Can you work these out from the drawing? Everything is in mm from the part's minimum corner. A direction names the side the tool comes from. Coordinates: 2 decimals unless noted, no trailing zeros. Order: outer loops, then holes, each group sorted by start corner. A loop starts at its lowest first (then second) coordinate and runs counter-clockwise, first axis right, second up. Notation, with made-up numbers: (80.5, 57.25) - (123.5, 57.25) arc R17 cw to (123.5, 61.25) - close; hole circle Ø10 at (15, 0.5). An arc over 180 degrees is marked (long way). Use a Markdown table: item, result. Add a question column.
(1) On a 3-axis mill with a long thin cutter (end or side, diameter ignored), from which of +Z, -Z, +X, -X, +Y, -Y can I reach the whole of each face in a straight line? I mean the marked faces 1 and 2. Say none if no direction works.
(2) I want a section at C-C (z = 7.5). State how many separate pieces and enclosed holes the cut face has, and give its area (3 significant figures).
(3) For pin 1 Ø3 at (y, z) = (44, 27.5) entering from +X; pin 2 Ø4 at (y, z) = (46, 9) entering from -X, each with a flat end and sliding along its axis, tell me the tip position at first contact or that it passes through.
(4) I want a section at D-D (x = 45). List the corners of the cut face in (y, z) for me, and give its area (3 significant figures).
(5) I want a section at A-A (y = 21.5). List the corners of the cut face in (x, z) for me.
(6) We'd pull the mould along Z, two halves only. Please class the marked faces 3, 4 and 5: pulls with the +Z half, pulls with the -Z half, needs draft (parallel to the pull), parting line crosses it, or undercut.
(7) I want a section at B-B (x = 23.5). List the corners of the cut face in (y, z) for me.
(8) If I drill on L1, parallel to Y at x = 8.5, z = 15.5; L2, parallel to Z at x = 20, y = 7; L3, parallel to X at y = 30, z = 31, over which ranges is the centre line in solid material (lowest first)? Write a range as [from, to].
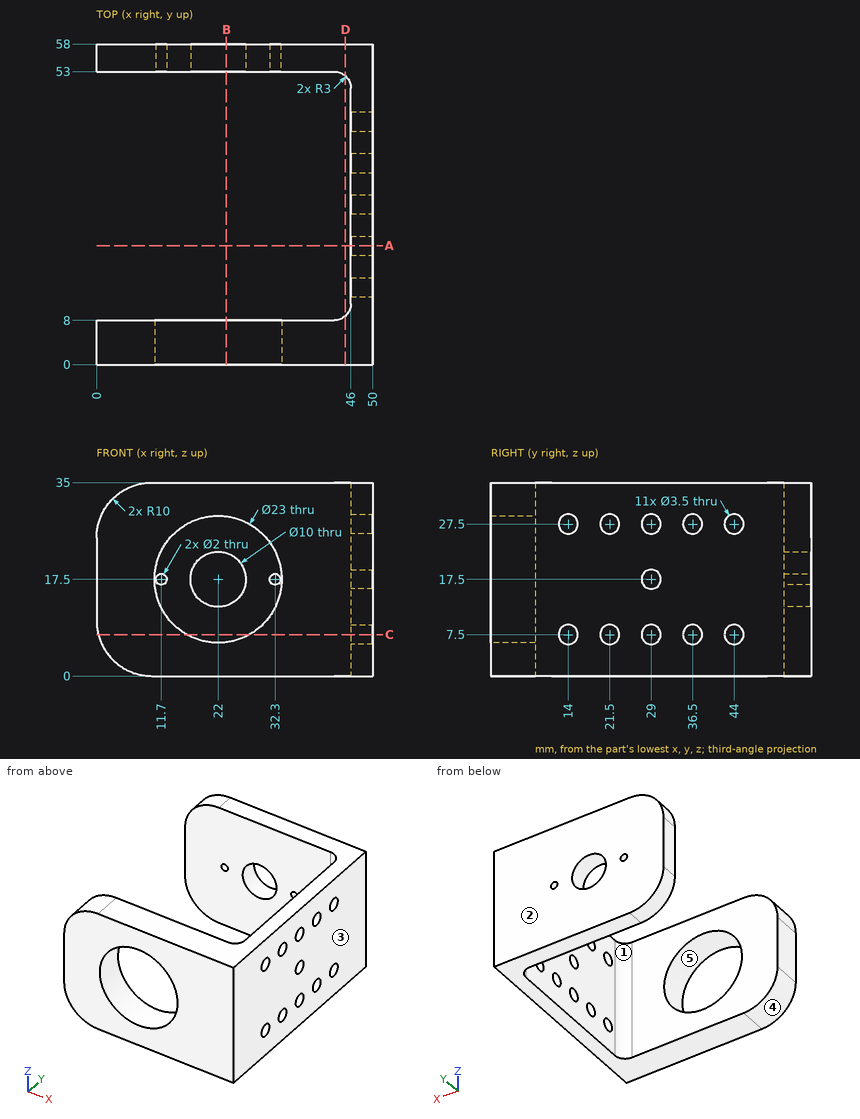
Answers follow:
| question | item | result |
|---|---|---|
| 1 | face 1 | +Z, -Z, -X |
| 1 | face 2 | +Z, -Z, +X, -X, +Y |
| 2 | separate pieces | 7 |
| 2 | enclosed holes | 0 |
| 2 | area | 669 mm² |
| 3 | pin 1 | passes through |
| 3 | pin 2 | stops at x = 46 |
| 4 | outline | (0, 0) - (8.76, 0) - (8.76, 35) - (0, 35) - close; (52.24, 0) - (58, 0) - (58, 35) - (52.24, 35) - close |
| 4 | area | 508 mm² |
| 5 | outline | (46, 0) - (50, 0) - (50, 5.75) - (46, 5.75) - close; (46, 9.25) - (50, 9.25) - (50, 25.75) - (46, 25.75) - close; (46, 29.25) - (50, 29.25) - (50, 35) - (46, 35) - close |
| 6 | face 3 | needs draft |
| 6 | face 4 | pulls with the -Z half |
| 6 | face 5 | undercut |
| 7 | outline | (0, 0) - (8, 0) - (8, 6.1) - (0, 6.1) - close; (0, 28.9) - (8, 28.9) - (8, 35) - (0, 35) - close; (53, 0) - (58, 0) - (58, 12.73) - (53, 12.73) - close; (53, 22.27) - (58, 22.27) - (58, 35) - (53, 35) - close |
| 8 | L1 | y = [0, 8], [53, 58] |
| 8 | L2 | z = [0, 6.18], [28.82, 35] |
| 8 | L3 | x = [46, 50] |
